Design review of the part shown in the three views and the two pictorial views. Dimensions are in mm from the part's minimum x, y and z. A direction names the side the tool comes from. Round coordinates to 2 decimals unless told otherwise and drop trailing zeros. Order: outer loops, then holes, each group sorted by start corner. A loop starts at its lowest first (then second) coordinate and runs counter-clockwise, first axis right, second up. Notation, with made-up numbers: (46, 83) - (81, 83) arc R26 cw to (81, 100) - close; hole circle Ø7 at (-16.75, 74.25). An arc over 180 degrees is marked (long way). Use CSV: the item, a comma, the result in double quotes.
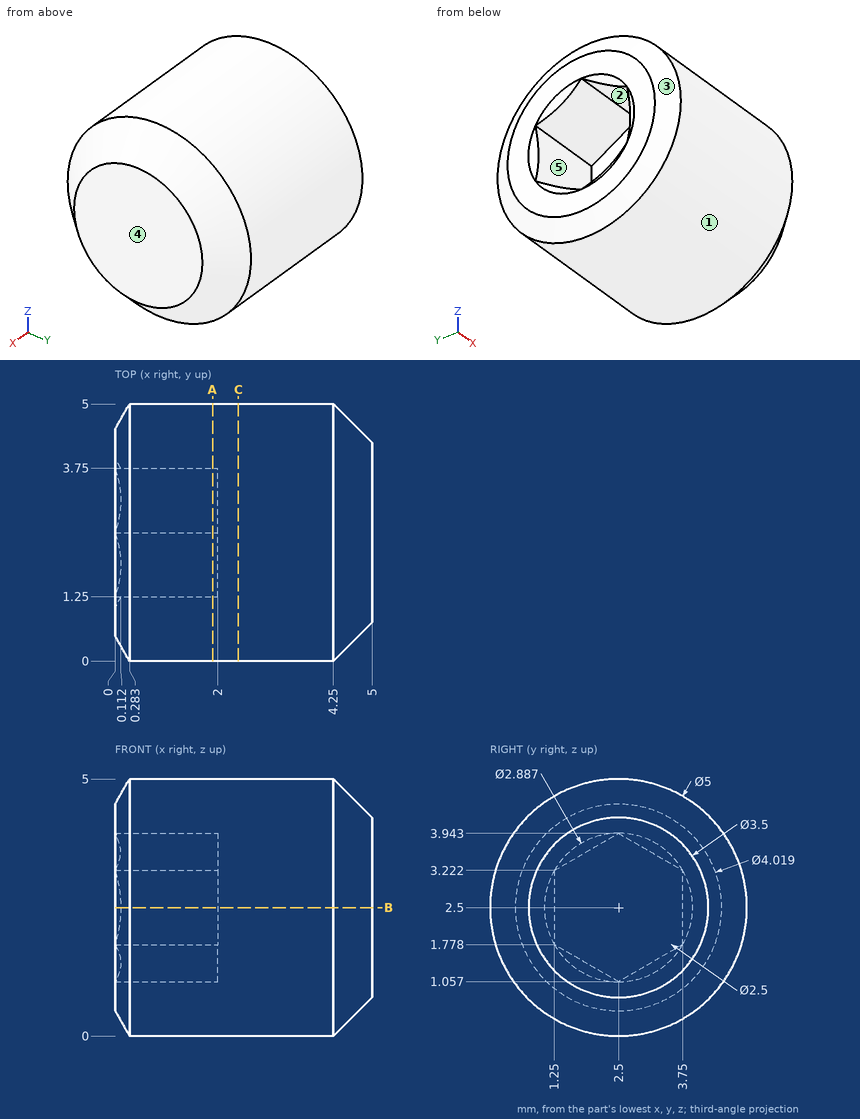
1) The part is to be moulded in two halves that separate along Y. For the marked faces 3, 4 and 5, say which applies: +Y half, -Y half, draft (parallel to the pull), parting line (faces both ways), or undercut.
Data:
face 3,"parting line"
face 4,"draft"
face 5,"undercut"
2) For the marked faces 1 and 2, list the 3-axis set-ups (+Z, -Z, +X, -X, +Y, -Y) from which the entire face can be reached by the end or side of a thin tool; tool diameter is ignored.
Data:
face 1,"+X, -X"
face 2,"-X"
3) We need section C-C (x = 2.4). Give the boundary of the cut face in (y, z).
Data:
outline,"circle Ø5 at (2.5, 2.5)"
4) We need section A-A (x = 1.9). Give the boundary of the cut face in (y, z).
Data:
outline,"circle Ø5 at (2.5, 2.5); hole (1.25, 1.78) - (2.5, 1.06) - (3.75, 1.78) - (3.75, 3.22) - (2.5, 3.94) - (1.25, 3.22) - close"
5) We need section B-B (z = 2.5). Give the boundary of the cut face in (x, y).
Data:
outline,"(0, 0.49) - (0.28, 0) - (4.25, 0) - (5, 0.75) - (5, 4.25) - (4.25, 5) - (0.28, 5) - (0, 4.51) - (0, 3.94) - (0.11, 3.75) - (2, 3.75) - (2, 1.25) - (0.11, 1.25) - (0, 1.06) - close"
6) To check wall thickness, follow L1, parallel to X at y = 1.4, z = 2.25; L2, parallel to Y at x = 0.55, z = 1.6 (1 decimal); L3, parallel to Z at x = 0.4, y = 1.95 (1 decimal). State the ranges of each line that lie inside material, in increasing order. Write a range as from..to.
Data:
L1,"x = 2..5"
L2,"y = 0.2..1.6, 3.4..4.8"
L3,"z = 0.1..1.4, 3.6..4.9"
7) Insertion check: pin 1 Ø1 at (x, y) = (2.5, 1) entering from -Z. The pin has a flat end and moves straight along its axis. Give the tip position at first contact, or say it passes through.
Data:
pin 1,"stops at z = 0.21"
